```python
from build123d import *

# Parameters (mm, degrees)
EXTRUDE_1_DEPTH     = 30
CUT_EXTRUDE_1_REACH = 43.003
SKETCH_2_W          = 12
SKETCH_2_H          = 20


with BuildPart() as part:
    # 草图1 → 凸台-拉伸1 (new body)
    with BuildSketch(Plane.XY):
        with BuildLine():
            Line((12.5, 10.5), (12.5, -10.5))
            ThreePointArc((12.5, -10.5), (11.914213562, -11.914213562), (10.5, -12.5))
            Line((10.5, -12.5), (-10.5, -12.5))
            ThreePointArc((-10.5, -12.5), (-11.914213562, -11.914213562), (-12.5, -10.5))
            Line((-12.5, -10.5), (-12.5, 10.5))
            ThreePointArc((-12.5, 10.5), (-11.914213562, 11.914213562), (-10.5, 12.5))
            Line((-10.5, 12.5), (10.5, 12.5))
            ThreePointArc((10.5, 12.5), (11.914213562, 11.914213562), (12.5, 10.5))
        make_face()
        with BuildLine():
            Line((-9, 11), (9, 11))
            ThreePointArc((9, 11), (10.414213562, 10.414213562), (11, 9))
            Line((11, 9), (11, -9))
            ThreePointArc((11, -9), (10.414213562, -10.414213562), (9, -11))
            Line((9, -11), (-9, -11))
            ThreePointArc((-9, -11), (-10.414213562, -10.414213562), (-11, -9))
            Line((-11, -9), (-11, 9))
            ThreePointArc((-11, 9), (-10.414213562, 10.414213562), (-9, 11))
        make_face(mode=Mode.SUBTRACT)
    extrude(amount=EXTRUDE_1_DEPTH)

    # 草图2 → 切除-拉伸1 (cut, up to next)
    with BuildSketch(Plane(origin=(0, 12.5, 0), x_dir=(1, 0, 0), z_dir=(0, 1, 0)), mode=Mode.PRIVATE) as cut_extrude_1_sk1:
        with Locations((0, -10)):
            Rectangle(SKETCH_2_W, SKETCH_2_H)
    cut_extrude_1_tool1 = extrude(cut_extrude_1_sk1.sketch, amount=-CUT_EXTRUDE_1_REACH, mode=Mode.PRIVATE) & part.part
    add(cut_extrude_1_tool1.solids().sort_by_distance((0, 12.5, 10))[0], mode=Mode.SUBTRACT)


solid = part.part
```
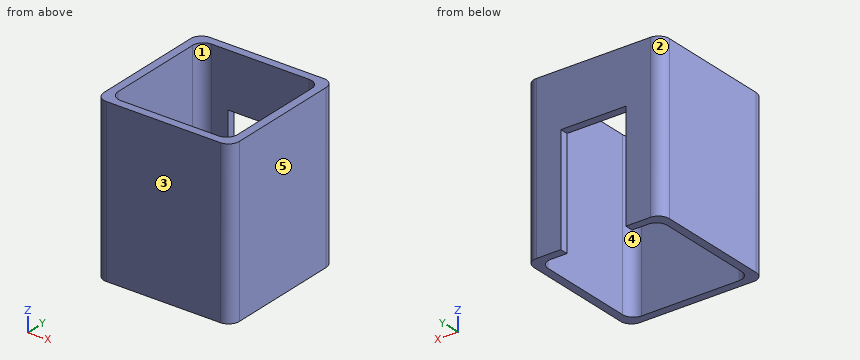
Model file for the job. Use its own axes, mm. Face numbers are marked on the shaded views. A direction names the side the tool comes from. Round coordinates to 2 decimals unless told otherwise and drop trailing zeros. Loops run counter-clockwise (first coordinate to the right, second up) from the corner with the lowest first, then second, coordinate; pieces in that order, holes last. Notation, with made-up numbers: M -16,-10 L 8,-10 A13 cw 8,-6 Z; hole C 27.25,67 d9. An arc over 180 degrees is marked long. Put each result on its own line as item: value. Start each with the question number.
Item 1: Drop flat-ended pins along their axis: P1, Ø5, axis at x = 3, z = 11, coming from the +Y side; P2, Ø4, axis at x = -8, y = -4, coming from the -Z side; P3, Ø1.6, axis at y = 12, z = 11, coming from the +X side; P4, Ø1.2, axis at x = -2.5, y = 12, coming from the -Z side. Give the stop position or say it passes through.
Item 2: 3-axis set-ups, long thin cutter, end or side, ignore diameter. For the marked faces 1 and 2: which of +Z, -Z, +X, -X, +Y, -Y reach the whole face in a straight line?
Item 3: Mould opens along Y. For the marked faces 3, 4 and 5 say: released by +Y, released by -Y, zero draft, split by the parting line, or undercut.
Item 4: Cut at B-B (y = 2). List the corners of the cut face in (x, z), then the cut area to 3 significant figures.
Item 5: Cut at C-C (z = 25). List the corners of the cut face in (x, y).
Item 6: Drill centre lines: line 1 along X through (y, z) = (-1.75, 25); line 2 along Y through (x, z) = (-3.5, 1.5). Where is each one in solid material? Low to high.
Item 7: Cut at D-D (z = 16). List the corners of the cut face in (x, y), then the cut area to 3 significant figures.
Item 8: Cut at A-A (x = -1.75). List the corners of the cut face in (y, z).
Answer block:
1. P1: y = -11
1. P2: through
1. P3: x = 12.37
1. P4: z = 20
2. face 1: +Z, -Z
2. face 2: +Z, -Z, -X, +Y
3. face 3: released by -Y
3. face 4: undercut
3. face 5: zero draft
4. outline: M -12.5,0 L -11,0 L -11,30 L -12.5,30 Z; M 11,0 L 12.5,0 L 12.5,30 L 11,30 Z
4. area: 90.0 mm2
5. outline: M -12.5,-10.5 A2 ccw -10.5,-12.5 L 10.5,-12.5 A2 ccw 12.5,-10.5 L 12.5,10.5 A2 ccw 10.5,12.5 L -10.5,12.5 A2 ccw -12.5,10.5 Z; hole M -11,-9 A2 ccw -9,-11 L 9,-11 A2 ccw 11,-9 L 11,9 A2 ccw 9,11 L -9,11 A2 ccw -11,9 Z
6. line 1: -12.5 to -11, 11 to 12.5
6. line 2: -12.5 to -11
7. outline: M -12.5,-10.5 A2 ccw -10.5,-12.5 L 10.5,-12.5 A2 ccw 12.5,-10.5 L 12.5,10.5 A2 ccw 10.5,12.5 L 6,12.5 L 6,11 L 9,11 A2 cw 11,9 L 11,-9 A2 cw 9,-11 L -9,-11 A2 cw -11,-9 L -11,9 A2 cw -9,11 L -6,11 L -6,12.5 L -10.5,12.5 A2 ccw -12.5,10.5 Z
7. area: 123 mm2
8. outline: M -12.5,0 L -11,0 L -11,30 L -12.5,30 Z; M 11,20 L 12.5,20 L 12.5,30 L 11,30 Z
